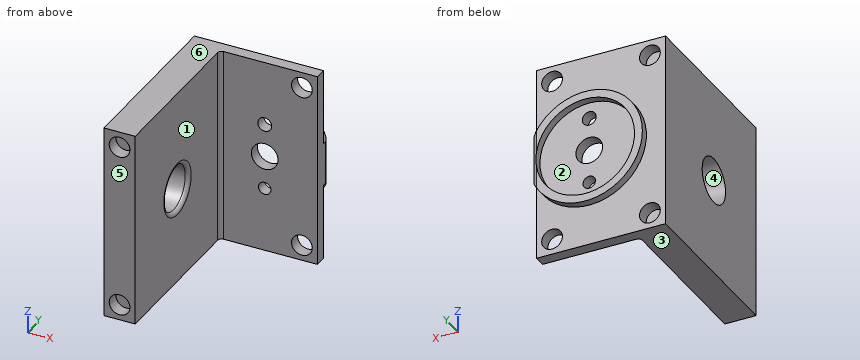
from build123d import *

# Parameters (mm, degrees)
SKETCH1_W           = 25
SKETCH1_H           = 50
SKETCH1_R           = 3.4
BOSS_EXTRUDE1_DEPTH = 3
SKETCH2_W           = 50
SKETCH2_H           = 3
BOSS_EXTRUDE2_DEPTH = 8
SKETCH3_W           = 8
SKETCH3_H           = 50
BOSS_EXTRUDE3_DEPTH = 42
SKETCH4_R           = 2.65
CUT_EXTRUDE1_DEPTH  = 3.3
SKETCH5_R           = 5.802370205
CUT_EXTRUDE2_DEPTH  = 9
FILLET2_R           = 1
SKETCH6_R           = 12.6
BOSS_EXTRUDE4_DEPTH = 2
FILLET3_R           = 1
FILLET4_R           = 1
SKETCH8_R           = 1.589780168
SKETCH8_R_2         = 1.777428262
CUT_EXTRUDE3_DEPTH  = 10


with BuildPart() as part:
    # Sketch1 → Boss-Extrude1 (new body)
    with BuildSketch(Plane(origin=(0, 0, 0), x_dir=(1, 0, 0), z_dir=(0, 1, 0))):
        with Locations((2.276951673, 11.384758364)):
            Rectangle(SKETCH1_W, SKETCH1_H)
        with Locations(Location((1.276951673, 11.384758364, 0), (0, 0, 270))):
            Circle(SKETCH1_R, mode=Mode.SUBTRACT)
    extrude(amount=BOSS_EXTRUDE1_DEPTH)

    # Sketch2 → Boss-Extrude2 (add)
    with BuildSketch(Plane.ZY.offset(10.223048327)):
        with Locations((-11.384758364, 1.5)):
            Rectangle(SKETCH2_W, SKETCH2_H)
    extrude(amount=BOSS_EXTRUDE2_DEPTH)

    # Sketch3 → Boss-Extrude3 (add)
    with BuildSketch(Plane.XZ):
        with Locations((-14.223048327, -11.384758364)):
            Rectangle(SKETCH3_W, SKETCH3_H)
    extrude(amount=BOSS_EXTRUDE3_DEPTH)

    # Sketch4 → Cut-Extrude1 (cut)
    with BuildSketch(Plane(origin=(0, 3, 0), x_dir=(1, 0, 0), z_dir=(0, 1, 0))):
        with Locations(Location((-14.223048327, 32.384758364, 0), (0, 0, 270))):
            Circle(SKETCH4_R)
        with Locations(Location((-14.223048327, -9.615241636, 0), (0, 0, 270))):
            Circle(SKETCH4_R)
    cut_extrude1 = extrude(amount=-CUT_EXTRUDE1_DEPTH, mode=Mode.SUBTRACT)

    # Mirror1: Cut-Extrude1 across plane
    add(cut_extrude1.mirror(Plane.ZX.offset(-19.5)), mode=Mode.SUBTRACT)

    # Sketch5 → Cut-Extrude2 (cut)
    with BuildSketch(Plane.ZY.offset(18.223048327)):
        with Locations((-11.836279124, -21)):
            Circle(SKETCH5_R)
    extrude(amount=-CUT_EXTRUDE2_DEPTH, mode=Mode.SUBTRACT)

    # Fillet2
    fillet2_edges = [part.edges().sort_by_distance(p)[0] for p in [
        (-10.223048327, -21, -17.638649329),
    ]]
    fillet(fillet2_edges, radius=FILLET2_R)

    # Mirror2: Cut-Extrude1 across plane
    add(cut_extrude1.mirror(Plane.ZY.offset(1.723048327)), mode=Mode.SUBTRACT)

    # Sketch6 → Boss-Extrude4 (add)
    with BuildSketch(Plane(origin=(0, 3, 0), x_dir=(1, 0, 0), z_dir=(0, 1, 0))):
        with BuildLine():
            Line((14.776951673, 5.825082115), (14.776951673, 16.944434614))
            ThreePointArc((14.776951673, 16.944434614), (-13.323048327, 11.384758364), (14.776951673, 5.825082115))
        make_face()
        with Locations(Location((1.276951673, 11.384758364, 0), (0, 0, 270))):
            Circle(SKETCH6_R, mode=Mode.SUBTRACT)
    extrude(amount=BOSS_EXTRUDE4_DEPTH)

    # Fillet3
    fillet3_edges = [part.edges().sort_by_distance(p)[0] for p in [
        (-10.223048327, 0, -11.384758364),
    ]]
    fillet(fillet3_edges, radius=FILLET3_R)

    # Fillet4
    # the kernel refuses this fillet: 1 mm, written as the material it takes off along each edge
    with BuildSketch(Plane(origin=(14.776951673, 5, -3.325082115), x_dir=(0, -1, 0), z_dir=(0, 0, -1))) as fillet4_piece_1:
        with BuildLine():
            CenterArc((FILLET4_R, FILLET4_R), FILLET4_R, 180, 90)
            Line((0, FILLET4_R), (0, 0))
            Line((0, 0), (FILLET4_R, 0))
        make_face()
    extrude(amount=16.119352499, mode=Mode.SUBTRACT)

    # Sketch8 → Cut-Extrude3 (cut)
    with BuildSketch(Plane(origin=(0, 3, 0), x_dir=(1, 0, 0), z_dir=(0, 1, 0))):
        with Locations(Location((1.276951673, 19.884758364, 0), (0, 0, 270))):
            Circle(SKETCH8_R)
        with Locations(Location((1.276951673, 2.884758364, 0), (0, 0, 270))):
            Circle(SKETCH8_R_2)
    extrude(amount=-CUT_EXTRUDE3_DEPTH, mode=Mode.SUBTRACT)


solid = part.part
Build history of the part. All positions in model axes, mm. Face numbers are marked on the shaded views. A direction names the side the tool comes from. Coordinates: 2 decimals unless noted, no trailing zeros. Order: outer loops, then holes, each group sorted by start corner. A loop starts at its lowest first (then second) coordinate and runs counter-clockwise, first axis right, second up. Notation, with made-up numbers: (31.25, 43) -> (85.25, 43) arc R19 ccw to (85.25, 59) -> close; hole circle Ø4 at (-22.75, 87). An arc over 180 degrees is marked (long way). One line per item, written item: value.
(1) Slice it at A-A, the plane y = -21. List the corners of the cut face in (x, z), plus the area to 3 significant figures.
Checked values:
outline: (-18.22, -36.38) -> (-10.22, -36.38) -> (-10.22, -18.64) arc R1 ccw to (-11.22, -17.64) -> (-18.22, -17.64) -> close; (-18.22, -6.03) -> (-11.22, -6.03) arc R1 ccw to (-10.22, -5.03) -> (-10.22, 13.62) -> (-18.22, 13.62) -> close
area: 307 mm2
(2) Slice it at B-B, the plane z = -29. List the corners of the cut face in (x, y).
Checked values:
outline: (-18.22, -42) -> (-10.22, -42) -> (-10.22, -1) arc R1 cw to (-9.22, 0) -> (14.78, 0) -> (14.78, 3) -> (-18.22, 3) -> close
(3) Drop flat-ended pins along their axis: pin 1 Ø9 at (x, z) = (1.28, -11.38) entering from +Y; pin 2 Ø15 at (x, z) = (1.28, -11.38) entering from -Y; pin 3 Ø2.5 at (x, z) = (1.28, -19.88) entering from +Y; pin 4 Ø3 at (x, z) = (-14.22, -32.38) entering from -Y. Give the stop position or say it passes through.
Checked values:
pin 1: y = 3
pin 2: y = 0
pin 3: through
pin 4: y = -38.7
(4) Probe line 1 (Y direction, x = -7, z = -27.5); line 2 (Y direction, x = -14, z = 9); line 3 (X direction, y = -7, z = -32). List the from-to ranges inside material, lowest first. Write a range as [from, to].
Checked values:
line 1: [0, 3]
line 2: [-38.7, -0.3]
line 3: [-18.22, -10.22]
(5) Mould opens along Y. For the marked faces 4, 5 and 6 say: pulls with the +Y half, pulls with the -Y half, needs draft (parallel to the pull), parting line crosses it, or undercut.
Checked values:
face 4: undercut
face 5: pulls with the -Y half
face 6: needs draft
(6) Tool access for the marked faces 1, 2 and 3: list every direction of +Z, -Z, +X, -X, +Y, -Y with a clear straight run to the whole face (end or side of a thin tool).
Checked values:
face 1: +Z, -Z, +X, -Y
face 2: +Y
face 3: -Z, +X, -X, +Y, -Y
(7) Slice it at C-C, the plane x = -1.5. List the corners of the cut face in (y, z).
Checked values:
outline: (0, -36.38) -> (3, -36.38) -> (3, -25.72) -> (5, -25.72) -> (5, -23.67) -> (3, -23.67) -> (3, -13.35) -> (0, -13.35) -> close; (0, -9.42) -> (3, -9.42) -> (3, 0.91) -> (5, 0.91) -> (5, 2.95) -> (3, 2.95) -> (3, 13.62) -> (0, 13.62) -> close
(8) Slice it at D-D, the plane z = -2.5. List the corners of the cut face in (x, y).
Checked values:
outline: (-18.22, -42) -> (-10.22, -42) -> (-10.22, -1) arc R1 cw to (-9.22, 0) -> (-0.46, 0) -> (-0.46, 3) -> (-7.66, 3) -> (-7.66, 5) -> (-10.31, 5) -> (-10.31, 3) -> (-18.22, 3) -> close; (3.01, 0) -> (14.78, 0) -> (14.78, 3) -> (12.86, 3) -> (12.86, 5) -> (10.21, 5) -> (10.21, 3) -> (3.01, 3) -> close
